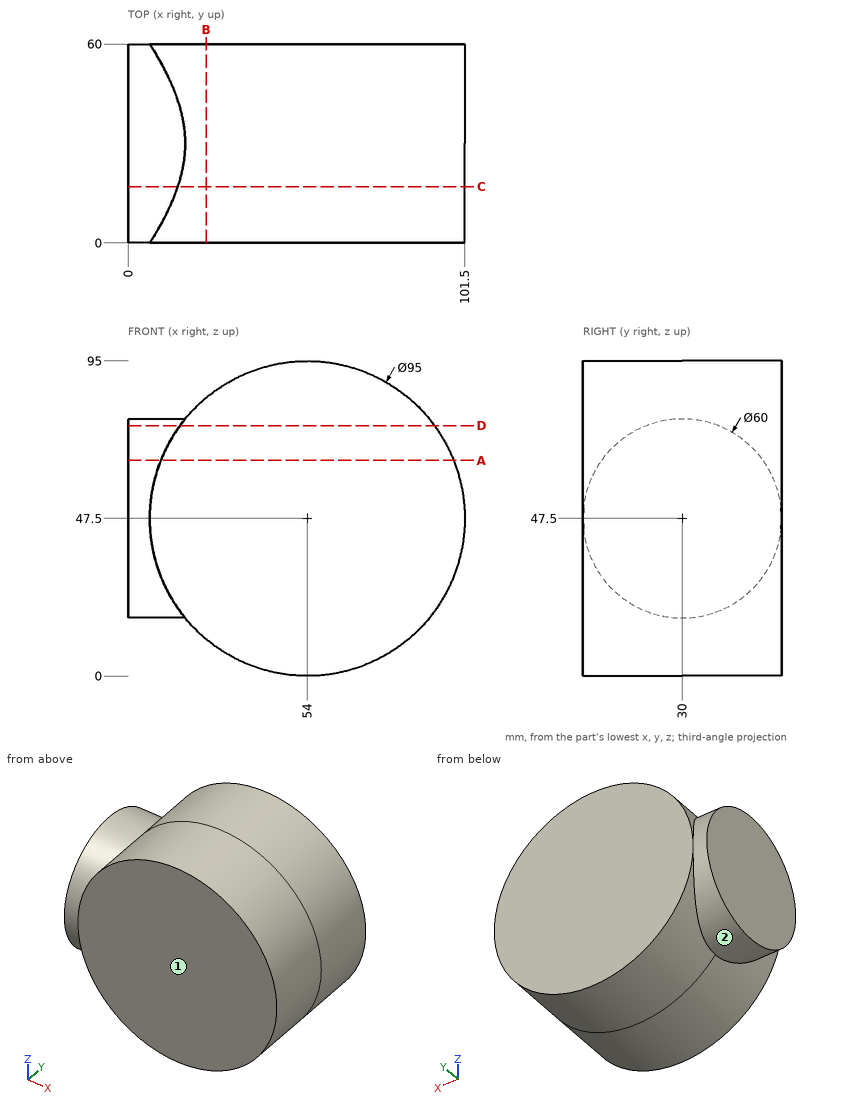
Design review of the part shown in the three views and the two pictorial views. Dimensions are in mm from the part's minimum x, y and z. A direction names the side the tool comes from. Coordinates: 2 decimals unless noted, no trailing zeros. Order: outer loops, then holes, each group sorted by start corner. A loop starts at its lowest first (then second) coordinate and runs counter-clockwise, first axis right, second up. Notation, with made-up numbers: (-7, 17) -> (3, 17) arc R21 ccw to (3, 45) -> close; hole circle Ø6 at (27.5, 69). An arc over 180 degrees is marked (long way). Use one line per item in the form item = value. Start each with the question number.
(1) Add section B-B on x = 23.5. State the section outline as (y, z) points, plus the area to 3 significant figures.
(2) Add section A-A on z = 65. State the section outline as (x, y) points.
(3) For the marked faces 1 and 2, list the 3-axis set-ups (+Z, -Z, +X, -X, +Y, -Y) from which the entire face can be reached by the end or side of a thin tool; tool diameter is ignored.
(4) Add section D-D on z = 75.5. State the section outline as (x, y) points, plus the area to 3 significant figures.
(5) Insertion check: pin 1 (5 mm diameter, centred on x = 69.5, y = 8, fed in from -Z); pin 2 (12 mm diameter, centred on x = 49, y = 32.5, fed in from +Z); pin 3 (1.5 mm diameter, centred on x = 66.5, y = 10.5, fed in from +Z). Each pin has a flat end and moves straight along its axis. Give the tip position at first contact, or say it passes through.
(6) For probe 1 along Z at (x, y) = (81, 24.5); probe 2 along Z at (x, y) = (41, 10); probe 3 along X at (y, z) = (22, 8.5), list the stretches that pass through material, from the lowest coordinate up.
(7) Add section C-C on y = 17. State the section outline as (x, z) points.
Answer block:
q1.outline = (0, 11.09) -> (60, 11.09) -> (60, 83.91) -> (0, 83.91) -> close
q1.area = 4,370 mm²
q2.outline = (0, 5.63) -> (9.84, 5.63) -> (9.84, 0) -> (98.16, 0) -> (98.16, 60) -> (9.84, 60) -> (9.84, 54.37) -> (0, 54.37) -> close
q3.face_1 = +Z, -Z, +X, -X, -Y
q3.face_2 = -X
q4.outline = (0, 19.23) -> (15.63, 19.23) -> (15.63, 0) -> (92.37, 0) -> (92.37, 60) -> (15.63, 60) -> (15.63, 40.77) -> (0, 40.77) -> close
q4.area = 4,940 mm²
q5.pin_1 = 1.81
q5.pin_2 = 95
q5.pin_3 = 93.52
q6.probe_1 = 8.42 to 86.58
q6.probe_2 = 1.81 to 93.19
q6.probe_3 = 26.88 to 81.12
q7.outline = (0, 20.46) -> (14.95, 20.46) arc R47.5 ccw (long way) to (14.95, 74.54) -> (0, 74.54) -> close
